from build123d import *

# Parameters (mm, degrees)
CROQUIS1_W                  = 248.76
CROQUIS1_H                  = 195
SALIENTE_EXTRUIR1_DEPTH     = 5
CROQUIS2_W                  = 48
CROQUIS2_H                  = 30
CROQUIS2_W_2                = 30
CORTAR_EXTRUIR1_DEPTH       = 2
CROQUIS3_R                  = 2.375
CORTAR_EXTRUIR2_DEPTH       = 10
CROQUIS4_R                  = 40
SALIENTE_EXTRUIR2_DEPTH     = 196.5
CROQUIS5_R                  = 12.5
CORTAR_EXTRUIR3_DEPTH       = 10
CROQUIS12_W                 = 12
CROQUIS12_H                 = 30
SALIENTE_EXTRUIR3_DEPTH     = 4
REDONDEO1_R                 = 10
REDONDEO2_R                 = 10
REDONDEO3_R                 = 10
CORTAR_EXTRUIR5_DEPTH       = 255.266033949
CORTAR_EXTRUIR5_DEPTH_BACK  = 255.266033949
CROQUIS13_R                 = 1.625
CORTAR_EXTRUIR7_DEPTH       = 2
CROQUIS16_R                 = 1.75
CORTAR_EXTRUIR9_DEPTH       = 20
CORTAR_EXTRUIR17_DEPTH      = 307.465597013
CORTAR_EXTRUIR17_DEPTH_BACK = 307.465597013
CROQUIS21_W                 = 105
CROQUIS21_H                 = 105
SALIENTE_EXTRUIR4_DEPTH     = 5
CHAFL_N1_SIZE               = 10


with BuildPart() as part:
    # Croquis1 → Saliente-Extruir1 (new body)
    with BuildSketch(Plane.XY):
        with Locations((7.088293187, 0.26268)):
            Rectangle(CROQUIS1_W, CROQUIS1_H)
    extrude(amount=SALIENTE_EXTRUIR1_DEPTH)

    # Croquis2 → Cortar-Extruir1 (cut)
    with BuildSketch(Plane.XY.offset(5)):
        with Locations((-93.291706813, -82.23732)):
            Rectangle(CROQUIS2_W, CROQUIS2_H)
        with Locations((116.468293187, 82.76268)):
            Rectangle(CROQUIS2_W_2, CROQUIS2_H)
        with Locations((116.468293187, -82.23732)):
            Rectangle(CROQUIS2_W_2, CROQUIS2_H)
        with Locations((-93.291706813, 82.76268)):
            Rectangle(CROQUIS2_W, CROQUIS2_H)
    extrude(amount=-CORTAR_EXTRUIR1_DEPTH, mode=Mode.SUBTRACT)

    # Croquis3 → Cortar-Extruir2 (cut)
    with BuildSketch(Plane.XY.offset(5)):
        with Locations((-93.291706813, 83.76268)):
            Circle(CROQUIS3_R)
        with Locations((-93.291706813, -83.23732)):
            Circle(CROQUIS3_R)
        with Locations((116.468293187, 83.76268)):
            Circle(CROQUIS3_R)
        with Locations((116.468293187, -83.23732)):
            Circle(CROQUIS3_R)
    extrude(amount=-CORTAR_EXTRUIR2_DEPTH, mode=Mode.SUBTRACT)

    # Croquis4 → Saliente-Extruir2 (add)
    with BuildSketch(Plane(origin=(0, 0, 0), x_dir=(-1, 0, 0), z_dir=(0, 0, -1))):
        with Locations(Location((55.101706813, 0.26268, 0), (0, 0, 180))):
            Circle(CROQUIS4_R)
    extrude(amount=SALIENTE_EXTRUIR2_DEPTH)

    # Croquis5 → Cortar-Extruir3 (cut)
    with BuildSketch(Plane(origin=(0, 0, 0), x_dir=(-1, 0, 0), z_dir=(0, 0, -1))):
        with Locations((-76.968293187, 0.26268)):
            Circle(CROQUIS5_R)
    extrude(amount=-CORTAR_EXTRUIR3_DEPTH, mode=Mode.SUBTRACT)

    # Croquis12 → Saliente-Extruir3 (add, symmetric)
    with BuildSketch(Plane(origin=(7.088293187, 0, 0), x_dir=(0, 0, -1), z_dir=(1, 0, 0))):
        with Locations((6, 82.76268)):
            Rectangle(CROQUIS12_W, CROQUIS12_H)
        with Locations((6, -82.23732)):
            Rectangle(CROQUIS12_W, CROQUIS12_H)
    extrude(amount=SALIENTE_EXTRUIR3_DEPTH, both=True)

    # Redondeo1
    redondeo1_edges = [part.edges().sort_by_distance(p)[0] for p in [
        (7.088293187, 67.76268, 0),
        (7.088293187, -67.23732, 0),
    ]]
    fillet(redondeo1_edges, radius=REDONDEO1_R)

    # Redondeo2
    redondeo2_edges = [part.edges().sort_by_distance(p)[0] for p in [
        (7.088293187, 67.76268, -12),
        (7.088293187, -67.23732, -12),
    ]]
    fillet(redondeo2_edges, radius=REDONDEO2_R)

    # Redondeo3
    redondeo3_edges = [part.edges().sort_by_distance(p)[0] for p in [
        (7.088293187, 97.76268, -12),
        (7.088293187, -97.23732, -12),
    ]]
    fillet(redondeo3_edges, radius=REDONDEO3_R)

    # Croquis13 → Cortar-Extruir5 (cut, two sides: drawn at the far end of the back side and taken through both)
    with BuildSketch(Plane(origin=(11.088293187, 0, 0), x_dir=(0, 0, -1), z_dir=(1, 0, 0)).offset(-CORTAR_EXTRUIR5_DEPTH_BACK)):
        with Locations(Location((6, 87.76268, 0), (0, 0, 90))):
            Circle(CROQUIS13_R)
        with Locations(Location((6, 77.76268, 0), (0, 0, 90))):
            Circle(CROQUIS13_R)
        with Locations(Location((6, -77.23732, 0), (0, 0, 90))):
            Circle(CROQUIS13_R)
        with Locations(Location((6, -87.23732, 0), (0, 0, 90))):
            Circle(CROQUIS13_R)
    extrude(amount=CORTAR_EXTRUIR5_DEPTH + CORTAR_EXTRUIR5_DEPTH_BACK, mode=Mode.SUBTRACT)

    # Croquis15 → Cortar-Extruir7 (cut)
    with BuildSketch(Plane.XY.offset(5)):
        Polygon((111.468293187, 67.76268), (131.468293187, 67.76268), (131.468293187, -67.23732), (111.468293187, -67.23732), (111.468293187, -59.48732), (125.218293187, -59.48732), (125.218293187, 60.01268), (111.468293187, 60.01268), align=None)
    extrude(amount=-CORTAR_EXTRUIR7_DEPTH, mode=Mode.SUBTRACT)

    # Croquis16 → Cortar-Extruir9 (cut)
    with BuildSketch(Plane.XY.offset(5)):
        with Locations((-55.101706813, 20.26268)):
            Circle(CROQUIS16_R)
        with Locations((-35.101706813, 0.26268)):
            Circle(CROQUIS16_R)
        with Locations((-55.101706813, -19.73732)):
            Circle(CROQUIS16_R)
        with Locations((-75.101706813, 0.26268)):
            Circle(CROQUIS16_R)
    extrude(amount=-CORTAR_EXTRUIR9_DEPTH, mode=Mode.SUBTRACT)

    # Croquis20 → Cortar-Extruir17 (cut, two sides: drawn at the far end of the back side and taken through both)
    with BuildSketch(Plane.XZ.offset(97.23732).offset(-CORTAR_EXTRUIR17_DEPTH_BACK)):
        Polygon((-117.291706813, 10.531534682), (-117.291706813, 0), (3.088293187, 0), (3.088293187, -12), (11.088293187, -12), (11.088293187, 0), (131.468293187, 0), (131.468293187, 10.531534682), align=None)
    extrude(amount=CORTAR_EXTRUIR17_DEPTH + CORTAR_EXTRUIR17_DEPTH_BACK, mode=Mode.SUBTRACT)

    # Croquis21 → Saliente-Extruir4 (add)
    with BuildSketch(Plane(origin=(0, 0, -196.5), x_dir=(-1, 0, 0), z_dir=(0, 0, -1))):
        with Locations((54.583486428, 1.233156347)):
            Rectangle(CROQUIS21_W, CROQUIS21_H)
    extrude(amount=SALIENTE_EXTRUIR4_DEPTH)

    # Chaflán1
    chafl_n1_edges = [part.edges().sort_by_distance(p)[0] for p in [
        (-95.101706813, 0.26268, -196.5),
    ]]
    chamfer(chafl_n1_edges, length=CHAFL_N1_SIZE)


solid = part.part
Verification items for the finished model (mm, model axes). A direction names the side the tool comes from. Give positions to 0.01 mm unless a question says otherwise; leave off trailing zeros. Loops run counter-clockwise (first coordinate to the right, second up) from the corner with the lowest first, then second, coordinate; pieces in that order, holes last.
1) Set-up check for faces 1 (the cylindrical face through (-60.3, -39.4, -91.9)), 2 (the flat face through (-54, -51.267, -199)): record each of +Z, -Z, +X, -X, +Y, -Y from which the full face is reachable in a straight line by a thin tool's end or side.
2) Sectioned sample at A-A, the plane z = -117. Enter the section's corners in (x, y).
3) Thickness scan on line 1 along Z through (x, y) = (-17, -42.5); line 2 along Y through (x, z) = (-57, -83.5); line 3 along Y through (x, z) = (-35, -12.5). Record the ranges inside material, lowest first.
4) Depth check by flat-ended pin: pin 1 Ø1.5 at (y, z) = (37, -66.5) entering from -X; pin 2 Ø1 at (x, y) = (-75, 0.5) entering from +Z; pin 3 Ø10 at (y, z) = (-11, -30.5) entering from +X (3 decimals). Enter the tip coordinate at first touch or a pass-through.
Answers:
1. face 1: +Z
1. face 2: +Z, -Z, +X, -X, -Y
2. outline: circle Ø80 at (-55.1, 0.26)
3. line 1: z = -201.5 to -196.5
3. line 2: y = -39.69 to 40.22
3. line 3: y = -34.32 to -1.48, 2.01 to 34.84
4. pin 1: stops at x = -72.56
4. pin 2: stops at z = -15
4. pin 3: stops at x = -15.595
